```python
from build123d import *

# Parameters (mm, degrees)
F0_W     = 2.413
F0_H     = 2.54
F1_DEPTH = 2.54


with BuildPart() as f1:
    # F0 (on Front) → F1 (new body)
    with BuildSketch(Plane.XZ):
        Polygon((-44.497715, 19.128243), (-46.910715, 19.128243), (-46.910715, 6.428243), (-46.24188, 6.91544), (-46.24188, 18.49121), (-25.985625, 18.49121), (-25.985625, 6.91544), (-25.320715, 6.428243), (-25.320715, 19.128243), (-27.733715, 19.128243), align=None)
        with Locations((-45.704215, 20.398243)):
            Rectangle(F0_W, F0_H)
        with Locations((-26.527215, 20.398243)):
            Rectangle(F0_W, F0_H)
    extrude(amount=F1_DEPTH)


solid = f1.part
```
Part model, mm, in its own coordinate system. A direction names the side the tool comes from. Round coordinates to 2 decimals unless told otherwise and drop trailing zeros. Loops run counter-clockwise (first coordinate to the right, second up) from the corner with the lowest first, then second, coordinate; pieces in that order, holes last.
Item 1: Cut at C-C, the plane x = -27.25. Give the cut face in (y, z).
Item 2: Cut at B-B, the plane y = -1.15. Give the cut face in (x, z).
Item 3: 3-axis set-ups, long thin cutter, end or side, ignore diameter. For faces 5 (the face through (-46, -1, 21.668)), 6 (the face through (-25.986, -1, 13)), 7 (the face through (-27.734, -1, 20)): which of +Z, -Z, +X, -X, +Y, -Y reach the whole face in a straight line?
Item 4: Cut at A-A, the plane z = 12. Give the cut face in (x, y).
Item 5: Cut at D-D, the plane x = -36.5. Give the cut face in (y, z).
Item 6: Drop a flat-ended pin along its axis: P1, Ø0.8, axis at x = -32.5, y = -1, coming from the -Z side. Give the stop position or say it passes through.
Item 7: Mould opens along X. For faces 1 (the face through (-25.321, -1, 14)), 2 (the face through (-46.911, -1, 14)), 3 (the face through (-44.498, -1, 20)), 4 (the face through (-27, -1, 21.668)) say: +X half, -X half, draft (parallel to the pull), parting line (faces both ways), or undercut.
Item 8: Drill centre lines: line 1 (X direction, y = -1.2, z = 19.5); line 2 (X direction, y = -2.2, z = 17.75); line 3 (Z direction, x = -46, y = -0.7). Where is each one in solid material? Low to high.
A:
1. outline: (-2.54, 18.49) - (0, 18.49) - (0, 21.67) - (-2.54, 21.67) - close
2. outline: (-46.91, 6.43) - (-46.24, 6.92) - (-46.24, 18.49) - (-25.99, 18.49) - (-25.99, 6.92) - (-25.32, 6.43) - (-25.32, 21.67) - (-27.73, 21.67) - (-27.73, 19.13) - (-44.5, 19.13) - (-44.5, 21.67) - (-46.91, 21.67) - close
3. face 5: +Z, +X, -X, +Y, -Y
3. face 6: -Z, +Y, -Y
3. face 7: +Z, +Y, -Y
4. outline: (-46.91, -2.54) - (-46.24, -2.54) - (-46.24, 0) - (-46.91, 0) - close; (-25.99, -2.54) - (-25.32, -2.54) - (-25.32, 0) - (-25.99, 0) - close
5. outline: (-2.54, 18.49) - (0, 18.49) - (0, 19.13) - (-2.54, 19.13) - close
6. P1: stops at z = 18.49
7. face 1: +X half
7. face 2: -X half
7. face 3: undercut
7. face 4: draft
8. line 1: x = -46.91 to -44.5, -27.73 to -25.32
8. line 2: x = -46.91 to -46.24, -25.99 to -25.32
8. line 3: z = 18.49 to 21.67
